Read the model definition and answer for the solid it produces. Units are mm, in the model's axes. A direction names the side the tool comes from. Give positions to 0.01 mm unless a question says otherwise; leave off trailing zeros. Order: outer loops, then holes, each group sorted by start corner. A loop starts at its lowest first (then second) coordinate and runs counter-clockwise, first axis right, second up.
```python
from build123d import *

# Parameters (mm, degrees)
F0_W     = 50
F0_H     = 35
F0_R     = 0.5
F0_R_2   = 10
F0_R_3   = 5.5
F1_DEPTH = 7
F2_START = 2
F2_DEPTH = 3


with BuildPart() as f1:
    # F0 (on Top) → F1 (new body)
    with BuildSketch(Plane.XY):
        with Locations((-8.4370832344, 3.1877499125)):
            Rectangle(F0_W, F0_H)
        with Locations((-30.4370832344, -10.3122500875)):
            Circle(F0_R, mode=Mode.SUBTRACT)
        with Locations((-26.4370832344, -10.3122500875)):
            Circle(F0_R, mode=Mode.SUBTRACT)
        with Locations((-22.4370832344, -10.3122500875)):
            Circle(F0_R, mode=Mode.SUBTRACT)
        with Locations((-30.4370832344, -6.3122500875)):
            Circle(F0_R, mode=Mode.SUBTRACT)
        with Locations((-26.4370832344, -6.3122500875)):
            Circle(F0_R, mode=Mode.SUBTRACT)
        with Locations((-22.4370832344, -6.3122500875)):
            Circle(F0_R, mode=Mode.SUBTRACT)
        with Locations((-30.4370832344, -2.3122500875)):
            Circle(F0_R, mode=Mode.SUBTRACT)
        with Locations((-26.4370832344, -2.3122500875)):
            Circle(F0_R, mode=Mode.SUBTRACT)
        with Locations((-22.4370832344, -2.3122500875)):
            Circle(F0_R, mode=Mode.SUBTRACT)
        with Locations((-30.4370832344, 1.6877499125)):
            Circle(F0_R, mode=Mode.SUBTRACT)
        with Locations((-26.4370832344, 1.6877499125)):
            Circle(F0_R, mode=Mode.SUBTRACT)
        with Locations((5.5629167656, -10.3122500875)):
            Circle(F0_R, mode=Mode.SUBTRACT)
        with Locations((9.5629167656, -10.3122500875)):
            Circle(F0_R, mode=Mode.SUBTRACT)
        with Locations((13.5629167656, -10.3122500875)):
            Circle(F0_R, mode=Mode.SUBTRACT)
        with Locations((5.5629167656, -6.3122500875)):
            Circle(F0_R, mode=Mode.SUBTRACT)
        with Locations((9.5629167656, -6.3122500875)):
            Circle(F0_R, mode=Mode.SUBTRACT)
        with Locations((13.5629167656, -6.3122500875)):
            Circle(F0_R, mode=Mode.SUBTRACT)
        with Locations((-8.4370832344, 0.6877499125)):
            Circle(F0_R_2, mode=Mode.SUBTRACT)
        with Locations((5.5629167656, -2.3122500875)):
            Circle(F0_R, mode=Mode.SUBTRACT)
        with Locations((9.5629167656, -2.3122500875)):
            Circle(F0_R, mode=Mode.SUBTRACT)
        with Locations((13.5629167656, -2.3122500875)):
            Circle(F0_R, mode=Mode.SUBTRACT)
        with Locations((9.5629167656, 1.6877499125)):
            Circle(F0_R, mode=Mode.SUBTRACT)
        with Locations((13.5629167656, 1.6877499125)):
            Circle(F0_R, mode=Mode.SUBTRACT)
        with Locations((-30.4370832344, 5.6877499125)):
            Circle(F0_R, mode=Mode.SUBTRACT)
        with Locations((-26.4370832344, 5.6877499125)):
            Circle(F0_R, mode=Mode.SUBTRACT)
        with Locations((-22.4370832344, 5.6877499125)):
            Circle(F0_R, mode=Mode.SUBTRACT)
        with Locations((-30.4370832344, 9.6877499125)):
            Circle(F0_R, mode=Mode.SUBTRACT)
        with Locations((-26.4370832344, 9.6877499125)):
            Circle(F0_R, mode=Mode.SUBTRACT)
        with Locations((-22.4370832344, 9.6877499125)):
            Circle(F0_R, mode=Mode.SUBTRACT)
        with Locations((-30.4370832344, 13.6877499125)):
            Circle(F0_R, mode=Mode.SUBTRACT)
        with Locations((-26.4370832344, 13.6877499125)):
            Circle(F0_R, mode=Mode.SUBTRACT)
        with Locations((-22.4370832344, 13.6877499125)):
            Circle(F0_R, mode=Mode.SUBTRACT)
        with Locations((-30.4370832344, 17.6877499125)):
            Circle(F0_R, mode=Mode.SUBTRACT)
        with Locations((-26.4370832344, 17.6877499125)):
            Circle(F0_R, mode=Mode.SUBTRACT)
        with Locations((-22.4370832344, 17.6877499125)):
            Circle(F0_R, mode=Mode.SUBTRACT)
        with Locations((-18.4370832344, 13.6877499125)):
            Circle(F0_R, mode=Mode.SUBTRACT)
        with Locations((-14.4370832344, 13.6877499125)):
            Circle(F0_R, mode=Mode.SUBTRACT)
        with Locations((-10.4370832344, 13.6877499125)):
            Circle(F0_R, mode=Mode.SUBTRACT)
        with Locations((-18.4370832344, 17.6877499125)):
            Circle(F0_R, mode=Mode.SUBTRACT)
        with Locations((-14.4370832344, 17.6877499125)):
            Circle(F0_R, mode=Mode.SUBTRACT)
        with Locations((-10.4370832344, 17.6877499125)):
            Circle(F0_R, mode=Mode.SUBTRACT)
        with Locations((5.5629167656, 5.6877499125)):
            Circle(F0_R, mode=Mode.SUBTRACT)
        with Locations((9.5629167656, 5.6877499125)):
            Circle(F0_R, mode=Mode.SUBTRACT)
        with Locations((13.5629167656, 5.6877499125)):
            Circle(F0_R, mode=Mode.SUBTRACT)
        with Locations((5.5629167656, 9.6877499125)):
            Circle(F0_R, mode=Mode.SUBTRACT)
        with Locations((9.5629167656, 9.6877499125)):
            Circle(F0_R, mode=Mode.SUBTRACT)
        with Locations((13.5629167656, 9.6877499125)):
            Circle(F0_R, mode=Mode.SUBTRACT)
        with Locations((-6.4370832344, 13.6877499125)):
            Circle(F0_R, mode=Mode.SUBTRACT)
        with Locations((-2.4370832344, 13.6877499125)):
            Circle(F0_R, mode=Mode.SUBTRACT)
        with Locations((1.5629167656, 13.6877499125)):
            Circle(F0_R, mode=Mode.SUBTRACT)
        with Locations((-6.4370832344, 17.6877499125)):
            Circle(F0_R, mode=Mode.SUBTRACT)
        with Locations((-2.4370832344, 17.6877499125)):
            Circle(F0_R, mode=Mode.SUBTRACT)
        with Locations((1.5629167656, 17.6877499125)):
            Circle(F0_R, mode=Mode.SUBTRACT)
        with Locations((5.5629167656, 13.6877499125)):
            Circle(F0_R, mode=Mode.SUBTRACT)
        with Locations((9.5629167656, 13.6877499125)):
            Circle(F0_R, mode=Mode.SUBTRACT)
        with Locations((13.5629167656, 13.6877499125)):
            Circle(F0_R, mode=Mode.SUBTRACT)
        with Locations((5.5629167656, 17.6877499125)):
            Circle(F0_R, mode=Mode.SUBTRACT)
        with Locations((9.5629167656, 17.6877499125)):
            Circle(F0_R, mode=Mode.SUBTRACT)
        with Locations((13.5629167656, 17.6877499125)):
            Circle(F0_R, mode=Mode.SUBTRACT)
        with Locations((-8.4370832344, 0.6877499125)):
            Circle(F0_R_2)
        with Locations((-8.4370832344, 0.6877499125)):
            Circle(F0_R_3, mode=Mode.SUBTRACT)
    extrude(amount=F1_DEPTH)


with BuildPart() as f2:
    # F0 (on Top) → F2 (new body)
    with BuildSketch(Plane.XY.offset(F2_START)):
        with Locations((-8.4370832344, 0.6877499125)):
            Circle(F0_R_2)
        with Locations((-8.4370832344, 0.6877499125)):
            Circle(F0_R_3, mode=Mode.SUBTRACT)
    extrude(amount=F2_DEPTH)


with BuildPart() as f1_1:
    add(f1.part)

    # F3: cut F2
    add(f2.part, mode=Mode.SUBTRACT)


solid = f1_1.part
```
1) Given pin 1 (14.5 mm diameter, centred on x = -8.44, y = 0.69, fed in from -Z), flat-ended and moving along its own axis, determine where the tip first touches the part or whether it passes through.
Final values:
pin 1: stops at z = 0
2) The part is cut by section B-B on y = 0. Determine the outline of the cut face in (x, z), and give its area (3 significant figures).
Final values:
outline: (-33.44, 0) - (-13.89, 0) - (-13.89, 2) - (-18.41, 2) - (-18.41, 5) - (-13.89, 5) - (-13.89, 7) - (-33.44, 7) - close; (-2.98, 0) - (16.56, 0) - (16.56, 7) - (-2.98, 7) - (-2.98, 5) - (1.54, 5) - (1.54, 2) - (-2.98, 2) - close
area: 246 mm2
3) For a pull along X with two mould halves and no side action, classify faces 3 (the face through (9.063, 1.71, 3.451)), 4 (the face through (-9, 7, 7)), 5 (the face through (13.45, 13.2, 3.45)) as released by +X, released by -X, zero draft, split by the parting line, or undercut.
Final values:
face 3: undercut
face 4: zero draft
face 5: undercut
4) Consider L1, parallel to Y at x = -18.5, z = 4; L2, parallel to Z at x = -7.5, y = -7.5; L3, parallel to Y at x = -2, z = 2.5. Determine where each line is inside the solid, lowest interval first.
Final values:
L1: y = -14.31 to 13.19, 14.18 to 17.19, 18.18 to 20.69
L2: z = 0 to 2, 5 to 7
L3: y = -14.31 to -6.96, 8.34 to 13.44, 13.93 to 17.44, 17.93 to 20.69
5) A tool of negligible diameter and unlimited length cuts with its end or side. For faces 1 (the face through (-4, -4, 2)), 2 (the face through (-25.975, 9.496, 3.451)), from which of +Z, -Z, +X, -X, +Y, -Y can it reach the whole face along a straight path? Write none if from no direction.
Final values:
face 1: none
face 2: +Z, -Z
6) The part is cut by section C-C on z = 4. Count the separate pieces of the cut face and the enclosed holes in it, and give its area (3 significant figures).
Final values:
separate pieces: 1
enclosed holes: 59
area: 1,390 mm2
7) The part is cut by section A-A on x = -3.5. Determine the outline of the cut face in (y, z).
Final values:
outline: (-14.31, 0) - (-1.74, 0) - (-1.74, 2) - (-8.01, 2) - (-8.01, 5) - (-1.74, 5) - (-1.74, 7) - (-14.31, 7) - close; (3.11, 0) - (20.69, 0) - (20.69, 7) - (3.11, 7) - (3.11, 5) - (9.38, 5) - (9.38, 2) - (3.11, 2) - close
